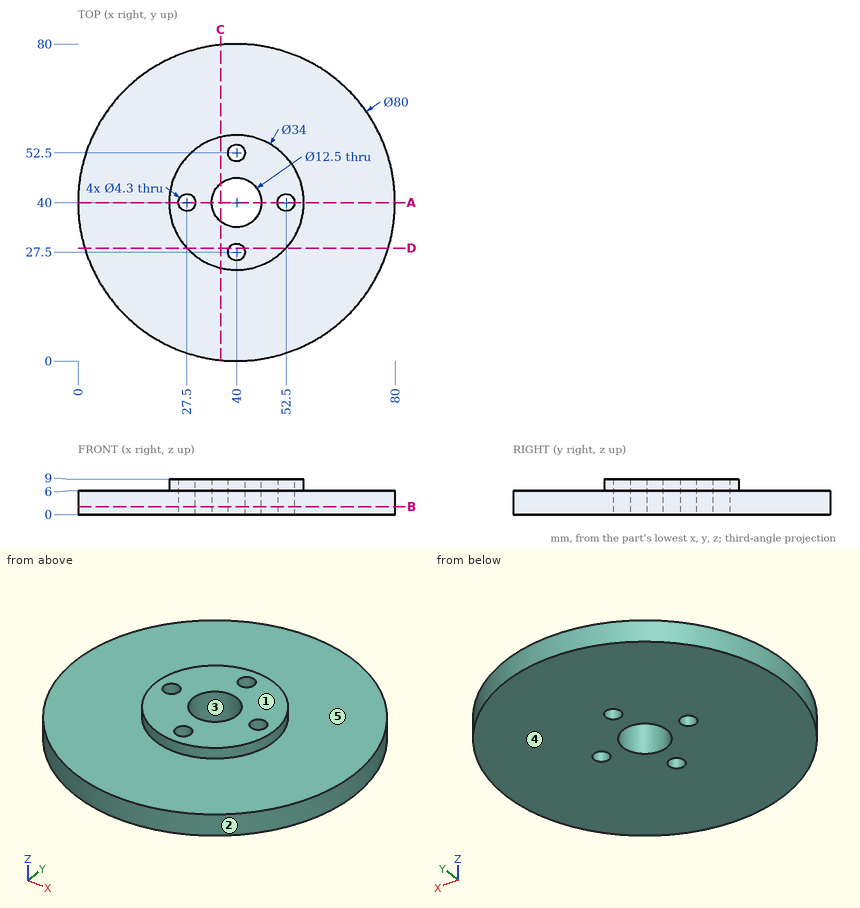
Part print with two shaded views. Sizes in mm from the minimum x, y, z corner. A direction names the side the tool comes from. Round coordinates to 2 decimals unless told otherwise and drop trailing zeros. Order: outer loops, then holes, each group sorted by start corner. A loop starts at its lowest first (then second) coordinate and runs counter-clockwise, first axis right, second up. Notation, with made-up numbers: M 43,68 L 48,68 A16 ccw 48,89 Z; hole C 50.25,69 d9. An arc over 180 degrees is marked long. Answer in a Markdown table with one row per item. Add a question column.
Q1. Pin check, flat tips, straight feed: pin 1 (2 mm diameter, centred on x = 71, z = 6.5, fed in from +Y); pin 2 (4 mm diameter, centred on x = 52, z = 4, fed in from -Y); pin 3 (5 mm diameter, centred on x = 62, z = 6.5, fed in from -Y). Stop position of each tip, or through.
Q2. Cut at C-C on x = 36. Give the cut face in (y, z).
Q3. Cut at B-B on z = 2. Give the cut face in (x, y).
Q4. Cut at D-D on y = 28.5. Give the cut face in (x, z), and give its area (3 significant figures).
Q5. Cut at A-A on y = 40. Give the cut face in (x, z), and give its area (3 significant figures).
Q6. Wall check: L1, parallel to Y at x = 40, z = 5; L2, parallel to Y at x = 40, z = 7.25; L3, parallel to Z at x = 58, y = 27.5. Give the ranges that are in metal, low to high. Write a range as from..to.
Q7. 3-axis set-ups, long thin cutter, end or side, ignore diameter. For the marked faces 4 and 5: which of +Z, -Z, +X, -X, +Y, -Y reach the whole face in a straight line?
Q8. Mould opens along Y. For the marked faces 1, 2 and 3 say: +Y half, -Y half, draft (parallel to the pull), parting line (faces both ways), or undercut.
Established:
| question | item | result |
|---|---|---|
| 1 | pin 1 | stops at y = 66.3 |
| 1 | pin 2 | stops at y = 1.27 |
| 1 | pin 3 | stops at y = 5.1 |
| 2 | outline | M 0.2,0 L 35.2,0 L 35.2,9 L 23.48,9 L 23.48,6 L 0.2,6 Z; M 44.8,0 L 79.8,0 L 79.8,6 L 56.52,6 L 56.52,9 L 44.8,9 Z |
| 3 | outline | C 40,40 d80; hole C 27.5,40 d4.3; hole C 40,40 d12.5; hole C 40,27.5 d4.3; hole C 40,52.5 d4.3; hole C 52.5,40 d4.3 |
| 4 | outline | M 1.69,0 L 38.1,0 L 38.1,9 L 27.48,9 L 27.48,6 L 1.69,6 Z; M 41.9,0 L 78.31,0 L 78.31,6 L 52.52,6 L 52.52,9 L 41.9,9 Z |
| 4 | area | 501 mm2 |
| 5 | outline | M 0,0 L 25.35,0 L 25.35,9 L 23,9 L 23,6 L 0,6 Z; M 29.65,0 L 33.75,0 L 33.75,9 L 29.65,9 Z; M 46.25,0 L 50.35,0 L 50.35,9 L 46.25,9 Z; M 54.65,0 L 80,0 L 80,6 L 57,6 L 57,9 L 54.65,9 Z |
| 5 | area | 392 mm2 |
| 6 | L1 | y = 0..25.35, 29.65..33.75, 46.25..50.35, 54.65..80 |
| 6 | L2 | y = 23..25.35, 29.65..33.75, 46.25..50.35, 54.65..57 |
| 6 | L3 | z = 0..6 |
| 7 | face 4 | -Z, +X, -X, +Y, -Y |
| 7 | face 5 | +Z |
| 8 | face 1 | draft |
| 8 | face 2 | parting line |
| 8 | face 3 | undercut |
